```python
from build123d import *

# Parameters (mm, degrees)
SKETCH1_R           = 36
SKETCH1_R_2         = 31
BOSS_EXTRUDE1_DEPTH = 1
SKETCH2_R           = 36
SKETCH2_R_2         = 34
BOSS_EXTRUDE2_DEPTH = 7
SKETCH3_R           = 36
SKETCH3_R_2         = 31
BOSS_EXTRUDE3_DEPTH = 1


with BuildPart() as part:
    # Sketch1 → Boss-Extrude1 (new body)
    with BuildSketch(Plane.XY):
        Circle(SKETCH1_R)
        Circle(SKETCH1_R_2, mode=Mode.SUBTRACT)
    extrude(amount=BOSS_EXTRUDE1_DEPTH)

    # Sketch2 → Boss-Extrude2 (add)
    with BuildSketch(Plane.XY.offset(1)):
        Circle(SKETCH2_R)
        Circle(SKETCH2_R_2, mode=Mode.SUBTRACT)
    extrude(amount=BOSS_EXTRUDE2_DEPTH)

    # Sketch3 → Boss-Extrude3 (add)
    with BuildSketch(Plane.XY.offset(8)):
        Circle(SKETCH3_R)
        Circle(SKETCH3_R_2, mode=Mode.SUBTRACT)
    extrude(amount=BOSS_EXTRUDE3_DEPTH)


solid = part.part
```
Part model, mm, in its own coordinate system. A direction names the side the tool comes from. Round coordinates to 2 decimals unless told otherwise and drop trailing zeros. Loops run counter-clockwise (first coordinate to the right, second up) from the corner with the lowest first, then second, coordinate; pieces in that order, holes last.
Item 1: 3-axis set-ups, long thin cutter, end or side, ignore diameter. For faces 4 (the face through (-4.036, 30.736, 0.493)), 5 (the face through (15, -28, 8)): which of +Z, -Z, +X, -X, +Y, -Y reach the whole face in a straight line?
Item 2: Mould opens along Y. For faces 1 (the face through (-4.686, 35.694, 4.437)), 2 (the face through (16, 27, 0)), 3 (the face through (18.28, 28.67, 4.45)) say: +Y half, -Y half, draft (parallel to the pull), parting line (faces both ways), or undercut.
Item 3: Drill centre lines: line 1 (Y direction, x = 0, z = 3.5); line 2 (Y direction, x = 0, z = 8.5). Where is each one in solid material? Low to high.
Item 4: Cut at A-A, the plane x = 0. Give the cut face in (y, z), then the cut area to 3 significant figures.
Item 5: Drop flat-ended pins along their axis: P1, Ø1.5, axis at y = 7.5, z = 2, coming from the -X side; P2, Ø2, axis at x = -1.5, y = 28.5, coming from the -Z side; P3, Ø4, axis at y = -8.5, z = 1.5, coming from the +X side; P4, Ø3, axis at x = 27, z = 7.5, coming from the -Y side. Give the stop position or say it passes through.
Item 6: Cut at C-C, the plane z = 6.5. Give the cut face in (x, y).
A:
1. face 4: +Z, -Z
1. face 5: none
2. face 1: parting line
2. face 2: draft
2. face 3: undercut
3. line 1: y = -36 to -34, 34 to 36
3. line 2: y = -36 to -31, 31 to 36
4. outline: (-36, 0) - (-31, 0) - (-31, 1) - (-34, 1) - (-34, 8) - (-31, 8) - (-31, 9) - (-36, 9) - close; (31, 0) - (36, 0) - (36, 9) - (31, 9) - (31, 8) - (34, 8) - (34, 1) - (31, 1) - close
4. area: 48.0 mm2
5. P1: stops at x = -35.36
5. P2: passes through
5. P3: stops at x = 35.41
5. P4: stops at y = -25.41
6. outline: circle Ø72 at (0, 0); hole circle Ø68 at (0, 0)
